Job drawing, mm, ordinate dimensions from the low corner. One solid piece. A direction names the side the tool comes from. Round coordinates to 2 decimals unless told otherwise and drop trailing zeros. Loops run counter-clockwise (first coordinate to the right, second up) from the corner with the lowest first, then second, coordinate; pieces in that order, holes last. Notation, with made-up numbers: M -20.75,-36 L 12.25,-36 A36 ccw 12.25,1 Z; hole C -29.5,50 d10. An arc over 180 degrees is marked long. Put each result on its own line as item: value. Start each with the question number.
1) Slice it at A-A on y = 33. Give the cut face in (x, z).
2) Probe line 1 along Z through (x, y) = (116.85, 7.5); line 2 along X through (y, z) = (13, 130); line 3 along Y through (x, z) = (51.5, 30). List the from-to ranges inside material, lowest first.
3) Slice it at C-C on z = 64. Give the cut face in (x, y).
4) Which spindle directions (+Z, -Z, +X, -X, +Y, -Y) get a long thin tool onto all of the face, cutting with end or side? Do the marked faces 1 and 2. Say none if no direction does.
5) Slice it at D-D on x = 94. Give the cut face in (y, z).
6) Drop flat-ended pins along their axis: pin 1 Ø3 at (x, z) = (112, 82) entering from -Y; pin 2 Ø2 at (y, z) = (9, 54.5) entering from -X. Give the stop position or say it passes through.
7) Pull direction Y, two halves, no side cores. Call the marked faces 3, 4, 5 and 6: +Y half, -Y half, draft (parallel to the pull), parting line (faces both ways), or undercut.
8) Slice it at B-B on x = 66. Give the cut face in (y, z).
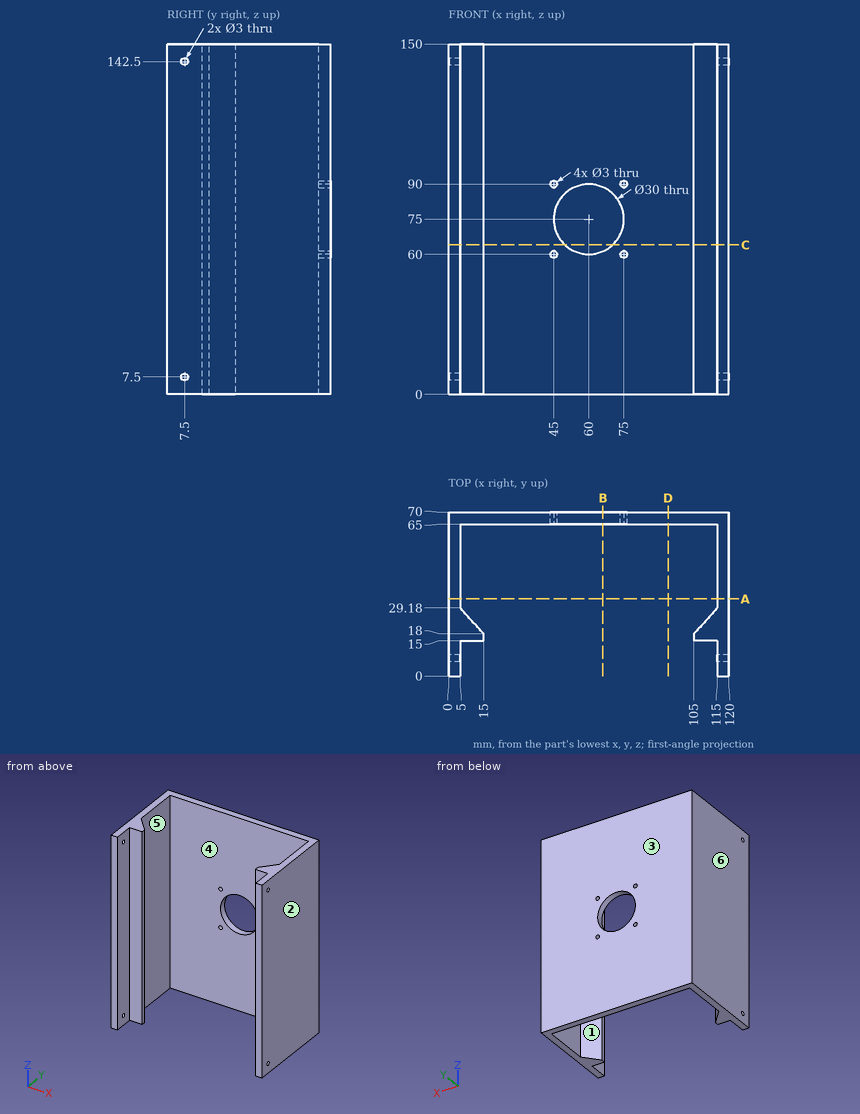
Recorded:
1. outline: M 0,0 L 5,0 L 5,150 L 0,150 Z; M 115,0 L 120,0 L 120,150 L 115,150 Z
2. line 1: z = 0 to 6, 9 to 141, 144 to 150
2. line 2: x = 0 to 5, 115 to 120
2. line 3: y = 65 to 70
3. outline: M 0,0 L 5,0 L 5,15 L 15,15 L 15,18 L 5,29.18 L 5,65 L 49.8,65 L 49.8,70 L 0,70 Z; M 70.2,65 L 115,65 L 115,29.18 L 105,18 L 105,15 L 115,15 L 115,0 L 120,0 L 120,70 L 70.2,70 Z
4. face 1: +Z, -Z
4. face 2: +Z, -Z, +X, +Y, -Y
5. outline: M 65,0 L 70,0 L 70,150 L 65,150 Z
6. pin 1: stops at y = 15
6. pin 2: stops at x = 0
7. face 3: +Y half
7. face 4: undercut
7. face 5: undercut
7. face 6: draft
8. outline: M 65,0 L 70,0 L 70,61.25 L 65,61.25 Z; M 65,88.75 L 70,88.75 L 70,150 L 65,150 Z
